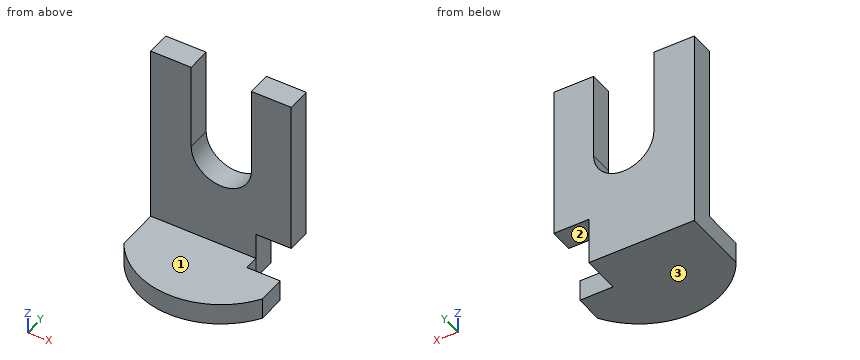
from build123d import *

# Parameters (mm, degrees)
F1_DEPTH = 25.4
F3_DEPTH = 22.606


with BuildPart() as f1:
    # F0 (on Front) → F1 (new body)
    with BuildSketch(Plane.XZ):
        with BuildLine():
            Line((4.654405, 101.662926), (-38.54106, 101.662926))
            Line((-38.54106, 101.662926), (-38.54106, -114.071727))
            Line((-38.54106, -114.071727), (73.815681, -114.071727))
            Line((73.815681, -114.071727), (73.815681, -63.353464))
            Line((73.815681, -63.353464), (111.429714, -63.353464))
            Line((111.429714, -63.353464), (111.429714, 101.662926))
            Line((111.429714, 101.662926), (68.962261, 101.662926))
            Line((68.962261, 101.662926), (68.962261, 8.962544))
            ThreePointArc((68.962261, 8.962544), (36.929212, -23.191613), (4.654405, 8.719872))
            Line((4.654405, 8.719872), (4.654405, 101.662926))
        make_face()
    extrude(amount=F1_DEPTH)

    # F2 (on face) → F3 (join)
    with BuildSketch(Plane(origin=(0, 0, -114.071727), x_dir=(1, 0, 0), z_dir=(0, 0, -1))):
        with BuildLine():
            Line((-38.54106, 71.035914), (-38.54106, 0))
            Line((-38.54106, 0), (73.70951, 0))
            Line((73.70951, 0), (73.70951, 40.798619))
            Line((73.70951, 40.798619), (109.369531, 40.798619))
            Line((109.369531, 40.798619), (109.369531, 71.035914))
            ThreePointArc((109.369531, 71.035914), (35.414236, 111.318798), (-38.54106, 71.035914))
        make_face()
    extrude(amount=-F3_DEPTH)


solid = f1.part
Input: part model. Units: mm. Frame: model coordinates. Face numbers are marked on the shaded views. A direction names the side the tool comes from. Give positions to 0.01 mm unless a question says otherwise; leave off trailing zeros. Write each loop counter-clockwise with the first axis right and the second up, starting at its lowest first coordinate (ties: lowest second). Pieces come first, ordered by that corner, then holes.
Q1. Material intervals for probe 1 along Y at (x, z) = (-4.5, 58); probe 2 along Z at (x, y) = (88, -9.5); probe 3 along X at (y, z) = (-10, -66.5), sorted ascending.
Q2. Section A-A, the plane z = 28. Output: boundary loops of the cut face in (x, y), plus the area to 3 significant figures.
Q3. Set-up query: the marked faces 1, 2 and 3. Return all of +Z, -Z, +X, -X, +Y, -Y with unobstructed straight access to the full face (end or side cutting, diameter ignored); none if empty.
Q4. Section B-B, the plane y = -23. Output: boundary loops of the cut face in (x, z), plus the area to 3 significant figures.
Q5. Section C-C, the plane x = 13. Output: boundary loops of the cut face in (y, z), plus the area to 3 significant figures.
Q6. Section D-D, the plane z = -80. Output: boundary loops of the cut face in (x, y).
Q7. First-contact query: P1, Ø18, axis at x = 92.5, z = -101.5, coming from the +Y side; P2, Ø2, axis at x = -17.5, y = -44.5, coming from the +Z side; P3, Ø6, axis at x = 68.5, z = 27.5, coming from the +Y side; P4, Ø17, axis at y = -34.5, z = -98, coming from the +X side. Flat tips, straight axial feed; report the tip coordinate or a pass-through.
Filled in:
1. probe 1: y = -25.4 to 0
1. probe 2: z = -63.35 to 101.66
1. probe 3: x = -38.54 to 73.82
2. outline: (-38.54, -25.4) - (4.65, -25.4) - (4.65, 0) - (-38.54, 0) - close; (68.96, -25.4) - (111.43, -25.4) - (111.43, 0) - (68.96, 0) - close
2. area: 2,180 mm2
3. face 1: +Z, +X, -X, -Y
3. face 2: -Z, +X, +Y, -Y
3. face 3: -Z, +X, -X, +Y, -Y
4. outline: (-38.54, -114.07) - (73.82, -114.07) - (73.82, -63.35) - (111.43, -63.35) - (111.43, 101.66) - (68.96, 101.66) - (68.96, 8.96) arc R32.15 cw to (4.65, 8.72) - (4.65, 101.66) - (-38.54, 101.66) - close
4. area: 22,900 mm2
5. outline: (-108.42, -114.07) - (0, -114.07) - (0, -12.65) - (-25.4, -12.65) - (-25.4, -91.47) - (-108.42, -91.47) - close
5. area: 4,450 mm2
6. outline: (-38.54, -25.4) - (73.82, -25.4) - (73.82, 0) - (-38.54, 0) - close
7. P1: stops at y = -40.8
7. P2: stops at z = -91.47
7. P3: stops at y = 0
7. P4: stops at x = 109.37
